from build123d import *

# Parameters (mm, degrees)
SKETCH1_W           = 25
SKETCH1_H           = 25
BOSS_EXTRUDE1_DEPTH = 20
CUT_EXTRUDE3_START  = -2.4
SKETCH2_W           = 22
SKETCH2_H           = 22
CUT_EXTRUDE3_DEPTH  = 15.2
CUT_EXTRUDE4_DEPTH  = 27.69269563
FILLET1_R           = 1
SKETCH5_R           = 2.5
CUT_EXTRUDE5_DEPTH  = 35.369317712
SKETCH6_R           = 2.5
CUT_EXTRUDE6_DEPTH  = 35.369317712


with BuildPart() as part:
    # Sketch1 → Boss-Extrude1 (new body)
    with BuildSketch(Plane.XY):
        Rectangle(SKETCH1_W, SKETCH1_H)
    extrude(amount=BOSS_EXTRUDE1_DEPTH)

    # Sketch2 → Cut-Extrude3 (cut)
    with BuildSketch(Plane.XY.offset(20).offset(CUT_EXTRUDE3_START)):
        with Locations((1.5, 1.5)):
            Rectangle(SKETCH2_W, SKETCH2_H)
    extrude(amount=-CUT_EXTRUDE3_DEPTH, mode=Mode.SUBTRACT)

    # Sketch3 → Cut-Extrude4 (cut, through all)
    with BuildSketch(Plane.XY.offset(20)):
        Polygon((-9.5, 3.166666667), (3.166666667, -9.5), (12.5, -9.5), (12.5, 12.5), (-9.5, 12.5), align=None)
    extrude(amount=-CUT_EXTRUDE4_DEPTH, mode=Mode.SUBTRACT)

    # Fillet1
    fillet1_edges = [part.edges().sort_by_distance(p)[0] for p in [
        (-12.5, 0, 20),
        (0, -12.5, 20),
        (12.5, -9.5, 10),
        (-9.5, 12.5, 10),
        (-3.166666667, -3.166666667, 17.6),
        (-11, 12.5, 0),
        (-3.166666667, -3.166666667, 2.4),
        (-3.166666667, -3.166666667, 0),
        (7.833333333, -9.5, 20),
        (7.833333333, -9.5, 0),
        (-3.166666667, -3.166666667, 20),
        (12.5, -11, 20),
        (0, -12.5, 0),
        (-12.5, 0, 0),
        (12.5, -11, 0),
        (12.5, -12.5, 10),
        (-12.5, -12.5, 10),
        (-12.5, 12.5, 10),
    ]]
    fillet(fillet1_edges, radius=FILLET1_R)

    # Sketch5 → Cut-Extrude5 (cut, through all)
    with BuildSketch(Plane.XZ.offset(12.5)):
        with Locations(Location((0, 10, 0), (0, 0, 270))):
            Circle(SKETCH5_R)
    extrude(amount=-CUT_EXTRUDE5_DEPTH, mode=Mode.SUBTRACT)

    # Sketch6 → Cut-Extrude6 (cut, through all)
    with BuildSketch(Plane.ZY.offset(12.5)):
        with Locations(Location((10, 0, 0), (0, 0, 270))):
            Circle(SKETCH6_R)
    extrude(amount=-CUT_EXTRUDE6_DEPTH, mode=Mode.SUBTRACT)


solid = part.part
Here's how the part is built. I have some questions about the finished solid (model axes, mm). A direction names the side the tool comes from. Coordinates: 2 decimals unless noted, no trailing zeros. Loops run counter-clockwise (first coordinate to the right, second up) from the corner with the lowest first, then second, coordinate; pieces in that order, holes last. Notation, with made-up numbers: (38.25, 76) -> (93.25, 76) arc R13 cw to (93.25, 82) -> close; hole circle Ø10 at (65.5, 52.5). An arc over 180 degrees is marked (long way). Use one line per item in the form item = value. Start each with the question number.
(1) If we section it at C-C (x = 8.75): Please give me the cut outline in (y, z), then the cut area to 3 significant figures.
(2) If we section it at A-A (z = 10): Please give me the cut outline in (x, y), then the cut area to 3 significant figures.
(3) If we section it at B-B (z = 16.25): Please give me the cut outline in (x, y), then the cut area to 3 significant figures.
(4) Please list where these lines run through material, in increasing order: line 1 along Z through (x, y) = (-10.5, 0); line 2 along X through (y, z) = (-11, 10); line 3 along Y through (x, z) = (-7.5, 17.5).
(5) Will these pins go through, and if not, where does the flat tip stop? pin 1 (6 mm diameter, centred on x = -7.5, z = 3, fed in from +Y); pin 2 (6 mm diameter, centred on y = 5, z = 8, fed in from +X); pin 3 (4 mm diameter, centred on x = 2, z = 11, fed in from +Y).
(6) If we section it at D-D (y = 4.25): Please give me the cut outline in (x, z).
(7) On a 3-axis mill with a long thin cutter (end or side, diameter ignored), from which of +Z, -Z, +X, -X, +Y, -Y can I reach the whole of each face in a straight line? I mean faces 1 (the face through (7.187, -9.801, 19.715)), 2 (the face through (7.187, -9.785, 0.301)), 3 (the face through (-3.28, -3.46, 2.1)). Say none if no direction works.
(8) We'd pull the mould along Z, two halves only. Please class faces 4 (the face through (-3.255, -3.078, 1.203)), 5 (the face through (-6, -6, 2.4)), 6 (the face through (-6, -6, 17.6)), 7 (the face through (12.199, -10.993, 19.715)): pulls with the +Z half, pulls with the -Z half, needs draft (parallel to the pull), parting line crosses it, or undercut.
Verdict:
q1.outline = (-12.5, 1) arc R1 ccw to (-11.5, 0) -> (-10.5, 0) arc R1 ccw to (-9.5, 1) -> (-9.5, 19) arc R1 ccw to (-10.5, 20) -> (-11.5, 20) arc R1 ccw to (-12.5, 19) -> close
q1.area = 59.1 mm²
q2.outline = (-12.5, -11.5) arc R1 ccw to (-11.5, -12.5) -> (-2.5, -12.5) -> (-2.5, -9.5) -> (-9.5, -9.5) -> (-9.5, -2.5) -> (-12.5, -2.5) -> close; (-12.5, 2.5) -> (-9.5, 2.5) -> (-9.5, 11.5) arc R1 ccw to (-10.5, 12.5) -> (-11.5, 12.5) arc R1 ccw to (-12.5, 11.5) -> close; (2.5, -12.5) -> (11.5, -12.5) arc R1 ccw to (12.5, -11.5) -> (12.5, -10.5) arc R1 ccw to (11.5, -9.5) -> (2.5, -9.5) -> close
q2.area = 110 mm²
q3.outline = (-12.5, -11.5) arc R1 ccw to (-11.5, -12.5) -> (11.5, -12.5) arc R1 ccw to (12.5, -11.5) -> (12.5, -10.5) arc R1 ccw to (11.5, -9.5) -> (-9.5, -9.5) -> (-9.5, 11.5) arc R1 ccw to (-10.5, 12.5) -> (-11.5, 12.5) arc R1 ccw to (-12.5, 11.5) -> close
q3.area = 140 mm²
q4.line_1 = 0 to 7.5, 12.5 to 20
q4.line_2 = -12.5 to -2.5, 2.5 to 12.5
q4.line_3 = -12.5 to -9.5
q5.pin_1 = 12.5
q5.pin_2 = -9.5
q5.pin_3 = -9.5
q6.outline = (-12.5, 1) arc R1 ccw to (-11.5, 0) -> (-9.5, 0) -> (-9.5, 20) -> (-11.5, 20) arc R1 ccw to (-12.5, 19) -> close
q7.face_1 = +Z, +X, +Y
q7.face_2 = -Z, +X, +Y
q7.face_3 = +X, +Y
q8.face_4 = needs draft
q8.face_5 = undercut
q8.face_6 = undercut
q8.face_7 = pulls with the +Z half
